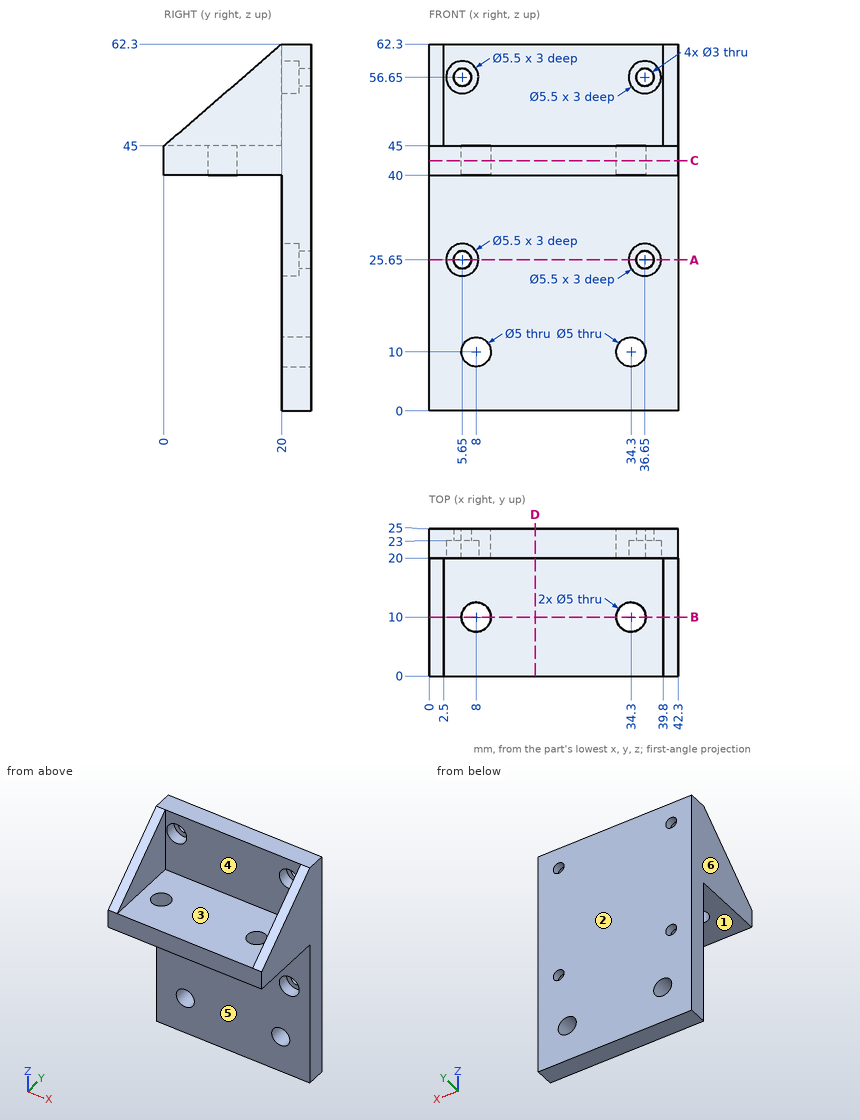
Verification items for this drawing (mm, ordinates from the low corner). A direction names the side the tool comes from. Give positions to 0.01 mm unless a question says otherwise; leave off trailing zeros. Order: outer loops, then holes, each group sorted by start corner. A loop starts at its lowest first (then second) coordinate and runs counter-clockwise, first axis right, second up.
1) Cross-section at A-A (z = 25.65). Record the boundary of the cut face in (x, y), then the cut area to 4 significant figures.
Results are:
outline: (0, 20) - (2.9, 20) - (2.9, 23) - (4.15, 23) - (4.15, 25) - (0, 25) - close; (7.15, 23) - (8.4, 23) - (8.4, 20) - (33.9, 20) - (33.9, 23) - (35.15, 23) - (35.15, 25) - (7.15, 25) - close; (38.15, 23) - (39.4, 23) - (39.4, 20) - (42.3, 20) - (42.3, 25) - (38.15, 25) - close
area: 166.5 mm2
2) Cross-section at C-C (z = 42.5). Record the boundary of the cut face in (x, y), then the cut area to 3 significant figures.
Results are:
outline: (0, 0) - (42.3, 0) - (42.3, 25) - (0, 25) - close; hole circle Ø5 at (8, 10); hole circle Ø5 at (34.3, 10)
area: 1,020 mm2
3) Gauge pin test, flat ends, axial feed: pin 1 (4 mm diameter, centred on x = 9, z = 29, fed in from -Y); pin 2 (2 mm diameter, centred on x = 10, y = 11.5, fed in from -Z); pin 3 (6 mm diameter, centred on x = 25, y = 7, fed in from +Z); pin 4 (12 mm diameter, centred on y = 10, z = 12.5, fed in from -X). Record the tip position at first contact, or that the pin passes through.
Results are:
pin 1: stops at y = 20
pin 2: stops at z = 40
pin 3: stops at z = 45
pin 4: passes through
4) Draft check along X on the marked faces 4, 5 and 6. Enter one of: released by +X, released by -X, zero draft, split by the parting line, or undercut.
Results are:
face 4: undercut
face 5: zero draft
face 6: released by -X
5) Cross-section at D-D (x = 18). Record the boundary of the cut face in (y, z).
Results are:
outline: (0, 40) - (20, 40) - (20, 0) - (25, 0) - (25, 62.3) - (20, 62.3) - (20, 45) - (0, 45) - close
6) Tool access check on the marked faces 1, 2 and 3. Record the directions out of +Z, -Z, +X, -X, +Y, -Y that give a thin tool (end or side, any length) a straight path to the whole face; none if there is none.
Results are:
face 1: -Z, +X, -X, -Y
face 2: +Z, -Z, +X, -X, +Y
face 3: +Z, -Y
7) Cross-section at B-B (y = 10). Record the boundary of the cut face in (x, z).
Results are:
outline: (0, 40) - (5.5, 40) - (5.5, 45) - (2.5, 45) - (2.5, 53.65) - (0, 53.65) - close; (10.5, 40) - (31.8, 40) - (31.8, 45) - (10.5, 45) - close; (36.8, 40) - (42.3, 40) - (42.3, 53.65) - (39.8, 53.65) - (39.8, 45) - (36.8, 45) - close
8) Material ranges on probe 1 along X at (y, z) = (22.3, 10); probe 2 along X at (y, z) = (22, 56.65); probe 3 along Y at (x, z) = (5.5, 17), recorded low to high.
Results are:
probe 1: x = 0 to 5.5, 10.5 to 31.8, 36.8 to 42.3
probe 2: x = 0 to 2.9, 8.4 to 33.9, 39.4 to 42.3
probe 3: y = 20 to 25
